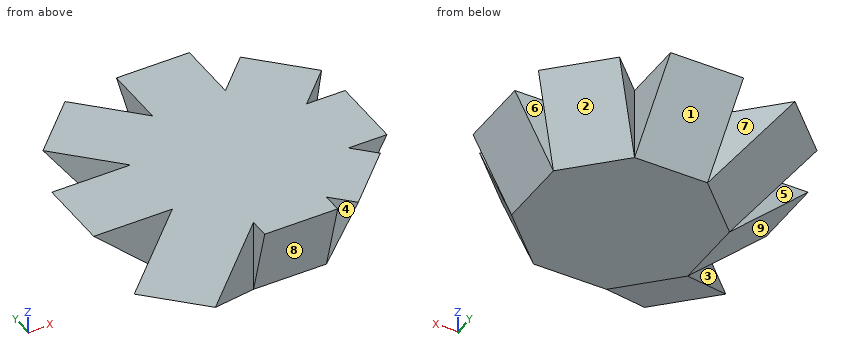
from build123d import *

# Parameters (mm, degrees)
F1_DEPTH  = 12.7
F5_DEPTH  = 6.35
F7_DEPTH  = 6.35
F9_DEPTH  = 6.35
F11_DEPTH = 6.35
F13_DEPTH = 6.35
F15_DEPTH = 6.35
F17_DEPTH = 6.35
F19_DEPTH = 6.35


with BuildPart() as f1:
    # F0 (on Top) → F1 (new body)
    with BuildSketch(Plane.XY):
        Polygon((6.35, -15.3302561211), (15.3302561211, -6.35), (15.3302561211, 6.35), (6.35, 15.3302561211), (-6.35, 15.3302561211), (-15.3302561211, 6.35), (-15.3302561211, -6.35), (-6.35, -15.3302561211), align=None)
    extrude(amount=-F1_DEPTH)

    # F4 (on Right) → F5 (join, symmetric)
    with BuildSketch(Plane.YZ):
        Polygon((-15.3302561211, -12.7), (-15.3302561211, 0), (-18.7332108649, 0), align=None)
    extrude(amount=F5_DEPTH, both=True)

    # F6 (on mid) → F7 (join, symmetric)
    with BuildSketch(Plane(origin=(0, 0, 0), x_dir=(0.7071067812, -0.7071067812, 0), z_dir=(-0.7071067812, -0.7071067812, 0))):
        Polygon((20.314638822, 0), (15.3302561211, 0), (15.3302561211, -12.7), align=None)
    extrude(amount=F7_DEPTH, both=True)

    # F8 (on Front) → F9 (join, symmetric)
    with BuildSketch(Plane.XZ):
        Polygon((22.0424020951, 0), (15.3302561211, 0), (15.3302561211, -12.7), align=None)
    extrude(amount=F9_DEPTH, both=True)

    # F10 (on mid) → F11 (join, symmetric)
    with BuildSketch(Plane(origin=(0, 0, 0), x_dir=(0.7071067812, 0.7071067812, 0), z_dir=(0.7071067812, -0.7071067812, 0))):
        Polygon((23.9889695097, 0), (15.3302561211, 0), (15.3302561211, -12.7), align=None)
    extrude(amount=F11_DEPTH, both=True)

    # F12 (on Right) → F13 (join, symmetric)
    with BuildSketch(Plane.YZ):
        Polygon((26.2594898514, 0), (15.3302561211, 0), (15.3302561211, -12.7), align=None)
    extrude(amount=F13_DEPTH, both=True)

    # F14 (on mid) → F15 (join, symmetric)
    with BuildSketch(Plane(origin=(0, 0, 0), x_dir=(0.7071067812, -0.7071067812, 0), z_dir=(-0.7071067812, -0.7071067812, 0))):
        Polygon((-15.3302561211, -12.7), (-15.3302561211, 0), (-29.0176009017, 0), align=None)
    extrude(amount=F15_DEPTH, both=True)

    # F16 (on Front) → F17 (join, symmetric)
    with BuildSketch(Plane.XZ):
        Polygon((-15.3302561211, -12.7), (-15.3302561211, 0), (-29.0176009017, 0), align=None)
    extrude(amount=F17_DEPTH, both=True)

    # F18 (on mid) → F19 (join, symmetric)
    with BuildSketch(Plane(origin=(0, 0, 0), x_dir=(0.7071067812, 0.7071067812, 0), z_dir=(0.7071067812, -0.7071067812, 0))):
        Polygon((-15.3302561211, -12.7), (-15.3302561211, 0), (-37.3273013772, 0), align=None)
    extrude(amount=F19_DEPTH, both=True)


solid = f1.part
Verification items for the finished model (mm, model axes). Face numbers are marked on the shaded views. A direction names the side the tool comes from. Give positions to 0.01 mm unless a question says otherwise; leave off trailing zeros. Write each loop counter-clockwise with the first axis right and the second up, starting at its lowest first coordinate (ties: lowest second). Pieces come first, ordered by that corner, then holes. Notation, with made-up numbers: M 35,-13 L 94,-13 A28 ccw 94,6 Z; hole C -36,-11.75 d2. An arc over 180 degrees is marked long. Put each result on its own line as item: value. Start each with the question number.
1. Section check D-D (y = -4). Record the cut outline in (x, z), and give its area (3 significant figures).
2. Section check A-A (x = -27). Record the cut outline in (y, z), and give its area (3 significant figures).
3. Go/stop test with flat-tipped pins: pin 1 Ø2 at (x, z) = (-3, -4.5) entering from -Y; pin 2 Ø1 at (y, z) = (5, -5) entering from -X; pin 3 Ø6.5 at (x, z) = (-24.5, -4.5) entering from +Y. Record where each tip stops, or that it passes through.
4. Section check C-C (z = -7.5). Record the cut outline in (x, y), and give its area (3 significant figures).
5. Scan lines: line 1 along Y through (x, z) = (-15.5, -11.5); line 2 along Y through (x, z) = (20.5, -2.5); line 3 along Y through (x, z) = (-17, -11). Record each from-to range of solid material in increasing order. Write a range as [from, to].
6. Set-up check for the marked faces 5, 6, 7, 8 and 9: record each of +Z, -Z, +X, -X, +Y, -Y from which the full face is reachable in a straight line by a thin tool's end or side.
7. Draft check along X on the marked faces 1, 2, 3 and 4. Enter one of: +X half, -X half, draft (parallel to the pull), parting line (faces both ways), or undercut.
8. Section check B-B (y = 20.5). Record the cut outline in (x, z), and give its area (3 significant figures).
Answer list:
1. outline: M -29.02,0 L -15.33,-12.7 L 15.33,-12.7 L 22.04,0 Z
1. area: 519 mm2
2. outline: M -25.79,0 L -18.02,-3.17 L -18.02,0 Z; M -6.35,-1.87 L 6.35,-1.87 L 6.35,0 L -6.35,0 Z
2. area: 36.1 mm2
3. pin 1: y = -17.8
3. pin 2: x = -24.17
3. pin 3: y = 15.6
4. outline: M -21.7,-12.72 L -12.72,-21.7 L -6.35,-15.33 L -6.35,-16.72 L 6.35,-16.72 L 6.35,-15.33 L 7.79,-16.77 L 16.77,-7.79 L 15.33,-6.35 L 18.08,-6.35 L 18.08,6.35 L 15.33,6.35 L 17.84,8.86 L 8.86,17.84 L 6.35,15.33 L 6.35,19.81 L -6.35,19.81 L -6.35,15.33 L -10.31,19.29 L -19.29,10.31 L -15.33,6.35 L -20.93,6.35 L -20.93,-6.35 L -15.33,-6.35 Z
4. area: 1,220 mm2
5. line 1: [-9.12, -6.52], [-6.35, 6.35], [6.52, 8.01]
5. line 2: [-6.35, 6.35]
5. line 3: [-8.84, -8.02], [-6.35, 6.35]
6. face 5: +Z, -Z, -X
6. face 6: +Z, -Z, +X
6. face 7: +Z, -Z, +Y
6. face 8: -Z, -Y
6. face 9: -Z, -X, +Y
7. face 1: draft
7. face 2: +X half
7. face 3: -X half
7. face 4: undercut
8. outline: M -20.54,0 L -11.52,-5.92 L -11.52,0 Z; M -6.35,-6.69 L 6.35,-6.69 L 6.35,0 L -6.35,0 Z; M 11.52,-1.98 L 13.43,0 L 11.52,0 Z
8. area: 114 mm2
